from build123d import *

# Parameters (mm, degrees)
SKETCH1_R           = 25.4
SKETCH1_R_2         = 20.32
BOSS_EXTRUDE1_DEPTH = 5.08
FILLET4_R           = 7.62
FILLET5_R           = 1.905
SKETCH2_R           = 1.5875


with BuildPart() as part:
    # Sketch1 → Boss-Extrude1 (new body)
    # profile 1 of 2: a face of its own
    with BuildSketch(Plane.XY):
        Circle(SKETCH1_R)
        Circle(SKETCH1_R_2, mode=Mode.SUBTRACT)
    # profile 2 of 2: a face of its own
    with BuildSketch(Plane.XY):
        with BuildLine():
            Line((2.54, -20.16062499), (2.54, -1.466469684))
            Line((2.54, -1.466469684), (18.729613398, 7.88060797))
            ThreePointArc((18.729613398, 7.88060797), (17.597636205, 10.16), (16.189613398, 12.280017021))
            Line((16.189613398, 12.280017021), (0, 2.932939367))
            Line((0, 2.932939367), (-16.189613398, 12.280017021))
            ThreePointArc((-16.189613398, 12.280017021), (-17.597636205, 10.16), (-18.729613398, 7.88060797))
            Line((-18.729613398, 7.88060797), (-2.54, -1.466469684))
            Line((-2.54, -1.466469684), (-2.54, -20.16062499))
            ThreePointArc((-2.54, -20.16062499), (0, -20.32), (2.54, -20.16062499))
        make_face()
        with BuildLine():
            ThreePointArc((1.414212148, 0.8763), (0, -1.6637), (-1.414212148, 0.8763))
            Line((-1.414212148, 0.8763), (1.414212148, 0.8763))
        make_face(mode=Mode.SUBTRACT)
    extrude(amount=BOSS_EXTRUDE1_DEPTH)

    # Fillet4
    fillet4_edges = [part.edges().sort_by_distance(p)[0] for p in [
        (2.54, -1.466469684, 2.54),
        (-2.54, -1.466469684, 2.54),
        (0, 2.932939367, 2.54),
    ]]
    fillet(fillet4_edges, radius=FILLET4_R)

    # Fillet5
    fillet5_edges = [part.edges().sort_by_distance(p)[0] for p in [
        (-17.597636205, -10.16, 5.08),
        (17.597636205, -10.16, 5.08),
        (-9.999806699, 8.706330457, 5.08),
        (9.999806699, 8.706330457, 5.08),
        (12.539806699, 4.306921406, 5.08),
        (2.54, -13.013251863, 5.08),
        (-2.54, -13.013251863, 5.08),
        (-12.539806699, 4.306921406, 5.08),
        (0, 4.11175747, 5.08),
        (3.560886423, -2.055878735, 5.08),
        (-3.560886423, -2.055878735, 5.08),
        (0, 20.32, 5.08),
    ]]
    fillet(fillet5_edges, radius=FILLET5_R)

    # Sketch2 → Cut-Revolve1 (revolve, cut)
    with BuildSketch(Plane(origin=(0, 0, 0), x_dir=(0, 0, -1), z_dir=(1, 0, 0)), mode=Mode.PRIVATE) as cut_revolve1_sk:
        with Locations((-2.54, 25.4)):
            Circle(SKETCH2_R)
    revolve(cut_revolve1_sk.sketch.rotate(Axis((0, 0, 5.08), (0, 0, -1)), 90), axis=Axis((0, 0, 5.08), (0, 0, -1)), mode=Mode.SUBTRACT)


solid = part.part
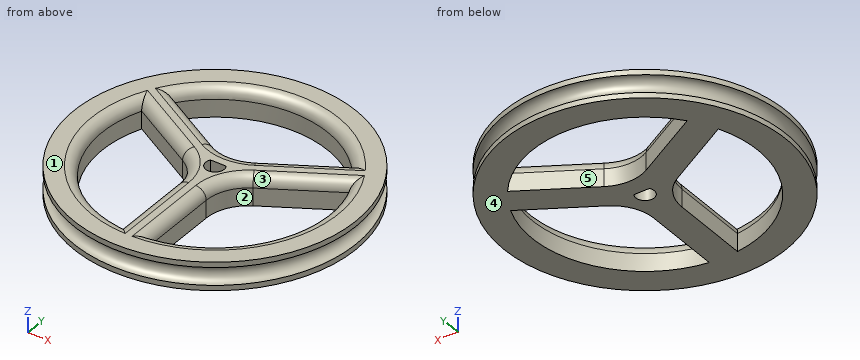
The model under review builds one solid part; all positions refer to its coordinate system, in mm. Face numbers are marked on the shaded views. A direction names the side the tool comes from. Coordinates: 2 decimals unless noted, no trailing zeros. Loops run counter-clockwise (first coordinate to the right, second up) from the corner with the lowest first, then second, coordinate; pieces in that order, holes last.
(1) Consider section A-A, the plane x = 0. Give the boundary of the cut face in (y, z) (1 decimal), plus the area to 3 significant figures.
Determined:
outline: (-25.4, 0) - (-1.7, 0) - (-1.7, 5.1) - (-25.4, 5.1) - (-25.4, 4.1) arc R1.6 cw to (-25.4, 1) - close; (0.9, 0) - (4.1, 0) - (4.1, 3.2) arc R1.9 ccw to (2.2, 5.1) - (0.9, 5.1) - close; (20.3, 0) - (25.4, 0) - (25.4, 1) arc R1.6 cw to (25.4, 4.1) - (25.4, 5.1) - (22.2, 5.1) arc R1.9 ccw to (20.3, 3.2) - close
area: 153 mm2
(2) Consider section C-C, the plane y = -9. Give the number of separate pieces and of enclosed holes in the cut face, plus the area to 3 significant figures.
Determined:
separate pieces: 3
enclosed holes: 0
area: 70.2 mm2
(3) Wall thickness on L1, parallel to Y at x = -1, z = 0.6; L2, parallel to Y at x = 15, z = 2.7; L3, parallel to X at y = -15.5, z = 2.7: over which ranges is each line inside the solid? List them lowest first.
Determined:
L1: y = -25.38 to -1.33, 0.88 to 4.18, 20.3 to 25.38
L2: y = -18.5 to -13.71, 5.73 to 11.59, 13.71 to 18.5
L3: x = -18.09 to -13.14, -2.54 to 2.54, 13.14 to 18.09
(4) Tool access review of the marked faces 1, 2 and 3: name each direction out of +Z, -Z, +X, -X, +Y, -Y from which nothing blocks a thin tool from reaching the whole face with its end or side.
Determined:
face 1: +Z, +X, -X, +Y, -Y
face 2: +Z, -Z
face 3: +Z
(5) Draft analysis for pull direction X (two halves, no side actions). For the marked faces 4 and 5, state which applies: +X half, -X half, draft (parallel to the pull), parting line (faces both ways), or undercut.
Determined:
face 4: draft
face 5: undercut
(6) Insertion check: P1, Ø1, axis at y = -12.5, z = 4.5, coming from the -X side; P2, Ø2, axis at x = -20, z = 3.5, coming from the +Y side; P3, Ø2.5, axis at x = -0.5, z = 3.5, coming from the -Y side; P4, Ø4, axis at x = 0, y = 0, coming from the -Z side. Each pin has a flat end and moves straight along its axis. Give the tip position at first contact, or say it passes through.
Determined:
P1: stops at x = -22.39
P2: stops at y = 16.6
P3: stops at y = -25.4
P4: stops at z = 0
(7) Consider section B-B, the plane z = 1.8. Give the boundary of the cut face in (x, y), plus the area to 3 significant figures.
Determined:
outline: circle Ø47.99 at (0, 0); hole (-18.73, 7.88) arc R20.32 ccw to (-2.54, -20.16) - (-2.54, -5.87) arc R7.62 ccw to (-6.35, 0.73) - close; hole (-16.19, 12.28) - (-3.81, 5.13) arc R7.62 ccw to (3.81, 5.13) - (16.19, 12.28) arc R20.32 ccw to start; hole (-1.41, 0.88) arc R1.66 ccw (long way) to (1.41, 0.88) - close; hole (2.54, -20.16) arc R20.32 ccw to (18.73, 7.88) - (6.35, 0.73) arc R7.62 ccw to (2.54, -5.87) - close
area: 812 mm2
